Could you check a few things on this model? Use its own coordinates, in mm. Face numbers are marked on the shaded views. A direction names the side the tool comes from. Give positions to 0.01 mm unless a question says otherwise; leave off trailing zeros. Write each loop counter-clockwise with the first axis right and the second up, starting at its lowest first coordinate (ties: lowest second). Pieces come first, ordered by that corner, then holes. Notation, with made-up numbers: (-16.5, 19) - (9.5, 19) arc R20 cw to (9.5, 55) - close; hole circle Ø1 at (36, 50.25). An arc over 180 degrees is marked (long way). Use one line per item in the form item = value.
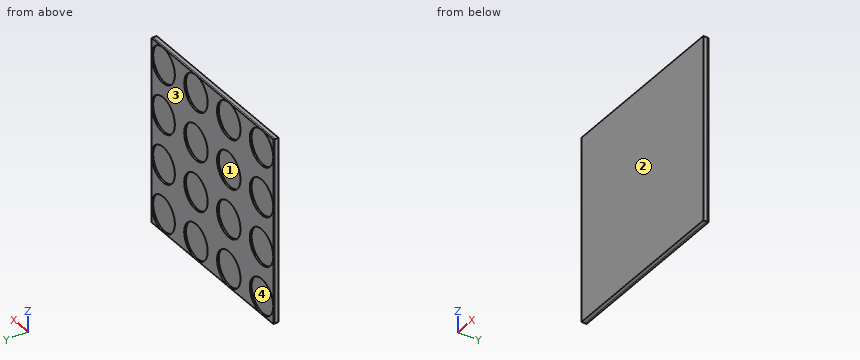
Autodesk Inventor part; units mm, degrees
ref_plane "YZ Plane" through (0, 0, 0) normal (1, 0, 0) x (0, 1, 0)
ref_plane "XZ Plane" through (0, 0, 0) normal (0, 1, 0) x (-1, 0, 0)
ref_plane "XY Plane" through (0, 0, 0) normal (0, 0, 1) x (1, 0, 0)
sketch "スケッチ1" plane through (0, 0, 0) normal (0, 1, 0) x (-1, 0, 0)
  line L0 (-52, 52) -> (52, 52)
  line L1 (52, 52) -> (52, -52)
  line L2 (52, -52) -> (-52, -52)
  line L3 (-52, -52) -> (-52, 52)
  point P0 (0, 0)
  dimension "d0" = 104
  dimension "d2" = 104
  dimension "d3" = 52
  dimension "d4" = 52
extrude "押し出し1" add sketch "スケッチ1" along normal blind 2
sketch "スケッチ2" plane through (0, 2, 0) normal (0, 1, 0) x (1, 0, 0)
  line L0 (-52, -52) -> (52, -52)
  line L1 (52, -52) -> (52, 52)
  line L2 (52, 52) -> (-52, 52)
  line L3 (-52, 52) -> (-52, -52)
  circle A0 centre (-42, -42) radius 10
  circle A1 centre (-14, -42) radius 10
  circle A2 centre (14, -42) radius 10
  circle A3 centre (-42, -14) radius 10
  circle A4 centre (-14, -14) radius 10
  circle A5 centre (14, -14) radius 10
  circle A6 centre (-42, 14) radius 10
  circle A7 centre (-14, 14) radius 10
  circle A8 centre (14, 14) radius 10
  circle A9 centre (42, -42) radius 10
  circle A10 centre (42, -14) radius 10
  circle A11 centre (42, 14) radius 10
  circle A12 centre (42, 42) radius 10
  circle A13 centre (14, 42) radius 10
  circle A14 centre (-14, 42) radius 10
  circle A15 centre (-42, 42) radius 10
  point P0 (0, 0)
  dimension "d7" = 20
  dimension "d43" = 28
  dimension "d44" = 28
  dimension "d45" = 28
  dimension "d46" = 10
  dimension "d47" = 10
  dimension "d48" = 10
  dimension "d49" = 10
  dimension "d50" = 10
  dimension "d51" = 10
  dimension "d52" = 28
  dimension "d53" = 28
  dimension "d54" = 28
  dimension "d55" = 28
  dimension "d56" = 28
  dimension "d57" = 28
  dimension "d58" = 28
  dimension "d59" = 28
  dimension "d60" = 28
  dimension "d61" = 28
  dimension "d62" = 28
  dimension "d63" = 10
  dimension "d64" = 10
  dimension "d65" = 28
  dimension "d66" = 28
  dimension "d67" = 28
  dimension "d68" = 28
  dimension "d69" = 28
  dimension "d70" = 28
  dimension "d71" = 28
  dimension "d72" = 28
  dimension "d73" = 28
  dimension "d74" = 28
extrude "押し出し2" add sketch "スケッチ2" along normal blind 1 contours L3 A0 L0 | A0 L3 A15 L2 A12 L1 A9 L0 | A9 L1 L0 | L3 L2 A15 | A12 L2 L1
properties part number "fai20_sikiita"
1. Which directions (+Z, -Z, +X, -X, +Y, -Y) give clear straight access to the entire face, cutting with the end or side of a thin tool? Please do the marked faces 3 and 4.
Response values:
face_3 = +Z, -Z, +X, -X, +Y
face_4 = +Y
2. Imagine slicing it at A-A, the plane x = -20. List the corners of the cut face in (y, z) for me.
Response values:
outline = (0, -52) - (3, -52) - (3, -50) - (2, -50) - (2, -34) - (3, -34) - (3, -22) - (2, -22) - (2, -6) - (3, -6) - (3, 6) - (2, 6) - (2, 22) - (3, 22) - (3, 34) - (2, 34) - (2, 50) - (3, 50) - (3, 52) - (0, 52) - close
3. Imagine slicing it at B-B, the plane z = 36. List the corners of the cut face in (x, y) for me, and give its area (3 significant figures).
Response values:
outline = (-52, 0) - (52, 0) - (52, 3) - (50, 3) - (50, 2) - (34, 2) - (34, 3) - (22, 3) - (22, 2) - (6, 2) - (6, 3) - (-6, 3) - (-6, 2) - (-22, 2) - (-22, 3) - (-34, 3) - (-34, 2) - (-50, 2) - (-50, 3) - (-52, 3) - close
area = 248 mm²
4. If I drill on line 1 (X direction, y = 2.4, z = -22.5); line 2 (X direction, y = 2.8, z = 35); line 3 (Y direction, x = -8, z = 14), over which ranges is the centre line in solid material (lowest first)? Write a range as from..to.
Response values:
line_1 = -52..-47.27, -36.73..-19.27, -8.73..8.73, 19.27..36.73, 47.27..52
line_2 = -52..-49.14, -34.86..-21.14, -6.86..6.86, 21.14..34.86, 49.14..52
line_3 = 0..2
5. For pin 1 (10 mm diameter, centred on x = 38.5, z = 13, fed in from +Y), with a flat end and sliding along its axis, tell me the tip position at first contact or that it passes through.
Response values:
pin_1 = 2
6. If we mould it in two halves opening along Z, with no side actions, what happens to the marked faces 1 and 2? For each: pulls with the +Z half, pulls with the -Z half, needs draft (parallel to the pull), parting line crosses it, or undercut.
Response values:
face_1 = undercut
face_2 = needs draft
